```python
from build123d import *

# Parameters (mm, degrees)
SKETCH_W     = 10
SKETCH_H     = 36.42
SKETCH_W_2   = 0.424
SKETCH_H_2   = 5
PAD_DEPTH    = 1
SKETCH001_W  = 5
SKETCH001_H  = 5
POCKET_DEPTH = 0.1


with BuildPart() as part:
    # Sketch → Pad (new body)
    with BuildSketch(Plane.XY):
        with Locations((5, 18.21)):
            Rectangle(SKETCH_W, SKETCH_H)
        with Locations((5, 14.9)):
            Rectangle(SKETCH_W_2, SKETCH_H_2, mode=Mode.SUBTRACT)
    extrude(amount=PAD_DEPTH)

    # Sketch001 (on Face10 of Pad) → Pocket (cut)
    with BuildSketch(Plane.XY.offset(1)):
        with Locations((5, 14.9)):
            Rectangle(SKETCH001_W, SKETCH001_H)
    extrude(amount=-POCKET_DEPTH, mode=Mode.SUBTRACT)


solid = part.part
```
Input: part model. Units: mm. Frame: model coordinates. A direction names the side the tool comes from. Round coordinates to 2 decimals unless told otherwise and drop trailing zeros.
1) Material intervals for line 1 (X direction, y = 12.5, z = 0.3); line 2 (X direction, y = 13.5, z = 0.95), sorted ascending.
Ans:
line 1: x = 0 to 4.79, 5.21 to 10
line 2: x = 0 to 2.5, 7.5 to 10
2) Set-up query: faces 1 (the flat face through (5.212, 14.9, 0.4)), 2 (the flat face through (4, 15, 0.9)), 3 (the flat face through (0, 18, 0.5)). Return all of +Z, -Z, +X, -X, +Y, -Y with unobstructed straight access to the full face (end or side cutting, diameter ignored); none if empty.
Ans:
face 1: +Z, -Z
face 2: +Z
face 3: +Z, -Z, -X, +Y, -Y
3) Pin query (flat end, axial travel): pin 1 (1.1 mm diameter, centred on x = 4, y = 14, fed in from +Z). Return the tip coordinate at first contact, or that it passes through.
Ans:
pin 1: stops at z = 0.9
4) Pull-direction query (Y, two-part tool) for faces 4 (the flat face through (4.9, 0, 0.5)), 5 (the flat face through (10, 18, 0.5)), 6 (the flat face through (4.788, 14.9, 0.4)); classes: released by +Y, released by -Y, zero draft, split by the parting line, or undercut.
Ans:
face 4: released by -Y
face 5: zero draft
face 6: undercut
